from build123d import *

# Parameters (mm, degrees)
F0_W     = 457.2
F0_H     = 254
F1_DEPTH = 25.4
F2_R     = 50.8
F3_R     = 12.7
F4_R     = 12.7


with BuildPart() as f1:
    # F0 (on Top) → F1 (new body)
    with BuildSketch(Plane.XY):
        with Locations((152.4, 0)):
            Rectangle(F0_W, F0_H)
    extrude(amount=-F1_DEPTH)

    # F2
    f2_edges = [f1.edges().sort_by_distance(p)[0] for p in [
        (-76.2, -127, -12.7),
        (381, -127, -12.7),
        (381, 127, -12.7),
        (-76.2, 127, -12.7),
    ]]
    fillet(f2_edges, radius=F2_R)

    # F3
    f3_edges = [f1.edges().sort_by_distance(p)[0] for p in [
        (152.4, -127, 0),
    ]]
    fillet(f3_edges, radius=F3_R)

    # F6: sweep along a path in F5
    with BuildLine(Plane.XZ) as f6_path:
        Line((0, 0), (0, 1473.2))
        ThreePointArc((0, 1473.2), (14.8789755157, 1509.1210244843), (50.8, 1524))
        Line((50.8, 1524), (254, 1524))
        ThreePointArc((254, 1524), (289.9210244843, 1509.1210244843), (304.8, 1473.2))
        Line((304.8, 1473.2), (304.8, 1371.6))
    # F4 (on face) → F6 (sweep)
    with BuildSketch(Plane.XY):
        Circle(F4_R)
    sweep(path=f6_path.line)


solid = f1.part
Could you check a few things on this model? Use its own coordinates, in mm. A direction names the side the tool comes from. Give positions to 0.01 mm unless a question says otherwise; leave off trailing zeros. Write each loop counter-clockwise with the first axis right and the second up, starting at its lowest first coordinate (ties: lowest second). Pieces come first, ordered by that corner, then holes. Notation, with made-up numbers: (-19, 52.5) -> (-7, 52.5) arc R25 cw to (-7, 80.5) -> close; hole circle Ø4 at (46, -2). An arc over 180 degrees is marked (long way). Answer as CSV lines item,"result". Start each with the question number.
(1) If we section it at C-C, the plane z = 1060: Write out the boundary of the cut face in (x, y), and give its area (3 significant figures).
(2) If we mould it in two halves opening along Z, with no side actions, what happens to faces 1 (the face through (153.822, 3.815, 1511.886)), 2 (the face through (-61.714, 111.724, -19.139)), 3 (the face through (149, 2, -25.4))? For each: +Z half, -Z half, draft (parallel to the pull), parting line (faces both ways), or undercut.
(3) Which directions (+Z, -Z, +X, -X, +Y, -Y) give clear straight access to the entire face, cutting with the end or side of a thin tool? Please do faces 4 (the face through (305, 0, 1371.6)), 5 (the face through (366.514, 111.724, -19.139)), 6 (the face through (292.686, 3.815, 1421.689)).
(4) Please list where these lines run through material, in increasing order: line 1 (Z direction, x = 359.5, y = -39); line 2 (Z direction, x = 285, y = -10); line 3 (X direction, y = -2, z = 397.5).
(5) If we section it at A-A, the plane z = 1387: Write out the boundary of the cut face in (x, y).
(6) I'm going to push a flat-ended pin straight in: pin 1 Ø1.5 at (x, y) = (317, 35) entering from +Z. Where does the tip first touch, or does it pass through?
(7) If we section it at B-B, the plane y = 58: Write out the boundary of the cut face in (x, z), and give its area (3 significant figures).
Answer list:
1,outline,"circle Ø25.4 at (0, 0)"
1,area,"507 mm^2"
2,face 1,"undercut"
2,face 2,"draft"
2,face 3,"-Z half"
3,face 4,"+X, +Y, -Y"
3,face 5,"+Z, -Z, +X, +Y"
3,face 6,"none"
4,line 1,"-25.4 to 0"
4,line 2,"-25.4 to 0, 1502.96 to 1522.96"
4,line 3,"-12.54 to 12.54"
5,outline,"circle Ø25.4 at (0, 0); circle Ø25.4 at (304.8, 0)"
6,pin 1,"z = 0"
7,outline,"(-76.2, -25.4) -> (381, -25.4) -> (381, -12.7) arc R12.7 ccw to (368.3, 0) -> (-63.5, 0) arc R12.7 ccw to (-76.2, -12.7) -> close"
7,area,"11,500 mm^2"
